```python
from build123d import *

# Parameters (mm, degrees)
SKETCH1_R           = 6
BOSS_EXTRUDE2_DEPTH = 12
BOSS_EXTRUDE3_DEPTH = 90
SKETCH4_R           = 6
CUT_EXTRUDE1_DEPTH  = 253.233216373


with BuildPart() as part:
    # Sketch1 → Boss-Extrude2 (new body)
    with BuildSketch(Plane(origin=(0, 0, 0), x_dir=(1, 0, 0), z_dir=(0, 1, 0))):
        with BuildLine():
            Line((350, 175), (350, 75))
            Line((350, 75), (238.484800354, 75))
            ThreePointArc((238.484800354, 75), (250, 0), (238.484800354, -75))
            Line((238.484800354, -75), (350, -75))
            Line((350, -75), (350, -175))
            Line((350, -175), (204.788011072, -143.394109088))
            Line((204.788011072, -143.394109088), (180.213449744, -126.186815997))
            ThreePointArc((180.213449744, -126.186815997), (220, 0), (180.213449744, 126.186815997))
            Line((180.213449744, 126.186815997), (204.788011072, 143.394109088))
            Line((204.788011072, 143.394109088), (350, 175))
        make_face()
        with Locations(Location((203.515969889, -117.5, 0), (0, 0, 270))):
            Circle(SKETCH1_R, mode=Mode.SUBTRACT)
        with Locations(Location((235, 0, 0), (0, 0, 270))):
            Circle(SKETCH1_R, mode=Mode.SUBTRACT)
        with Locations(Location((203.515969889, 117.5, 0), (0, 0, 270))):
            Circle(SKETCH1_R, mode=Mode.SUBTRACT)
    extrude(amount=BOSS_EXTRUDE2_DEPTH)

    # Sketch2 → Boss-Extrude3 (add)
    with BuildSketch(Plane(origin=(0, 0, 0), x_dir=(-1, 0, 0), z_dir=(0, -1, 0))):
        Polygon((-350, -175), (-350, -75), (-338, -75), (-338, -172.388158555), align=None)
        Polygon((-350, 75), (-350, 175), (-338, 172.388158555), (-338, 75), align=None)
    extrude(amount=BOSS_EXTRUDE3_DEPTH)

    # Sketch4 → Cut-Extrude1 (cut, through all)
    with BuildSketch(Plane.ZY.offset(-338)):
        with Locations((-150, -65)):
            Circle(SKETCH4_R)
        with Locations((-100, -65)):
            Circle(SKETCH4_R)
        with Locations((-125, -21.698729811)):
            Circle(SKETCH4_R)
        with Locations((150, -65)):
            Circle(SKETCH4_R)
        with Locations((125, -21.698729811)):
            Circle(SKETCH4_R)
        with Locations((100, -65)):
            Circle(SKETCH4_R)
    extrude(amount=-CUT_EXTRUDE1_DEPTH, mode=Mode.SUBTRACT)


solid = part.part
```
Check sheet for the modelled part. Datum: model origin and axes. Units: mm. A direction names the side the tool comes from. Give positions to 0.01 mm unless a question says otherwise; leave off trailing zeros. Write each loop counter-clockwise with the first axis right and the second up, starting at its lowest first coordinate (ties: lowest second). Pieces come first, ordered by that corner, then holes.
Item 1: Access from +Z, -Z, +X, -X, +Y, -Y to the whole of each face (thin tool, end or side, straight path). Record for faces 4 (the face through (338, -44, 123)), 5 (the face through (319, 3, 75)), 6 (the face through (343.916, -21.435, 119.006)).
Item 2: Scan lines: L1, parallel to Y at x = 345, z = -150; L2, parallel to Y at x = 344, z = 125; L3, parallel to Z at x = 341, y = -26. Record each from-to range of solid material in increasing order.
Item 3: Cross-section at D-D (x = 311). Enter the section's corners in (y, z).
Item 4: Cross-section at A-A (y = -65). Enter the section's corners in (x, z).
Item 5: Cross-section at C-C (y = -47). Enter the section's corners in (x, z), and give its area (3 significant figures).
Item 6: Gauge pin test, flat ends, axial feed: pin 1 (7 mm diameter, centred on y = -21.7, z = -125, fed in from +X); pin 2 (4 mm diameter, centred on x = 229, z = 44, fed in from -Y); pin 3 (15.5 mm diameter, centred on y = -65, z = -150, fed in from -X); pin 4 (15.5 mm diameter, centred on y = -65, z = -100, fed in from +X). Record the tip position at first contact, or that the pin passes through.
Item 7: Draft check along Z on faces 1 (the face through (240.95, 5.92, -0.78)), 2 (the face through (343.92, -68.65, -154.76)), 3 (the face through (344, -90, -126)). Enter one of: released by +Z, released by -Z, zero draft, split by the parting line, or undercut.
Item 8: Cross-section at B-B (z = -100). Enter the section's corners in (x, y), and give its area (3 significant figures).
Report:
1. face 4: +Z, -Z, -X, -Y
1. face 5: +X, +Y, -Y
1. face 6: +X, -X
2. L1: y = -90 to -71, -59 to 12
2. L2: y = -90 to -27.7, -15.7 to 12
2. L3: z = -173.04 to -129.18, -120.82 to -75, 75 to 120.82, 129.18 to 173.04
3. outline: (0, -166.51) - (12, -166.51) - (12, -75) - (0, -75) - close; (0, 75) - (12, 75) - (12, 166.51) - (0, 166.51) - close
4. outline: (338, -172.39) - (350, -175) - (350, -156) - (338, -156) - close; (338, -144) - (350, -144) - (350, -106) - (338, -106) - close; (338, -94) - (350, -94) - (350, -75) - (338, -75) - close; (338, 75) - (350, 75) - (350, 94) - (338, 94) - close; (338, 106) - (350, 106) - (350, 144) - (338, 144) - close; (338, 156) - (350, 156) - (350, 175) - (338, 172.39) - close
5. outline: (338, -172.39) - (350, -175) - (350, -75) - (338, -75) - close; (338, 75) - (350, 75) - (350, 175) - (338, 172.39) - close
5. area: 2,370 mm2
6. pin 1: passes through
6. pin 2: stops at y = 0
6. pin 3: stops at x = 338
6. pin 4: stops at x = 350
7. face 1: undercut
7. face 2: undercut
7. face 3: zero draft
8. outline: (195.96, 0) - (338, 0) - (338, -59) - (350, -59) - (350, 12) - (195.96, 12) - close; (338, -90) - (350, -90) - (350, -71) - (338, -71) - close
8. area: 2,780 mm2
